Read the model definition and answer for the solid it produces. Units are mm, in the model's axes. Face numbers are marked on the shaded views. A direction names the side the tool comes from. Round coordinates to 2 decimals unless told otherwise and drop trailing zeros. Order: outer loops, then holes, each group sorted by start corner. A loop starts at its lowest first (then second) coordinate and runs counter-clockwise, first axis right, second up. Notation, with made-up numbers: (43.5, 75.25) -> (50.5, 75.25) arc R22 cw to (50.5, 84.25) -> close; hole circle Ø7 at (67, 86.25). An arc over 180 degrees is marked (long way). Use a Markdown table: item, result. Add a question column.
1. Section D-D, the plane x = 54.5 is taken. Give the vertices of the cut face in (y, z).
2. Given pin 1 (1.5 mm diameter, centred on y = 22, z = 5.5, fed in from +X); pin 2 (3.5 mm diameter, centred on x = -59.24, z = 0, fed in from +Y); pin 3 (2.5 mm diameter, centred on y = 131.5, z = 23, fed in from +X); pin 4 (2 mm diameter, centred on x = 0, z = 59.24, fed in from -Y), each flat-ended and moving along its own axis, determine where each tip first touches the part or whether it passes through.
3. Consider L1, parallel to Z at x = 0, y = 1; L2, parallel to Y at x = -34, z = -12; L3, parallel to Z at x = -13, y = 45.5. Determine where each line is inside the solid, lowest interval first. Write a range as [from, to].
4. Section A-A, the plane x = 7 is taken. Give the vertices of the cut face in (y, z), then the cut area to 3 significant figures.
5. Section C-C, the plane z = 18.5 is taken. Give the vertices of the cut face in (x, y), then the cut area to 3 significant figures.
6. Section B-B, the plane y = 11.5 is taken. Give the vertices of the cut face in (x, z).
7. For the marked faces 1 and 2, determine the directions among +Z, -Z, +X, -X, +Y, -Y from which every point of the face is accessible in a straight line to the end or side of a thin tool.
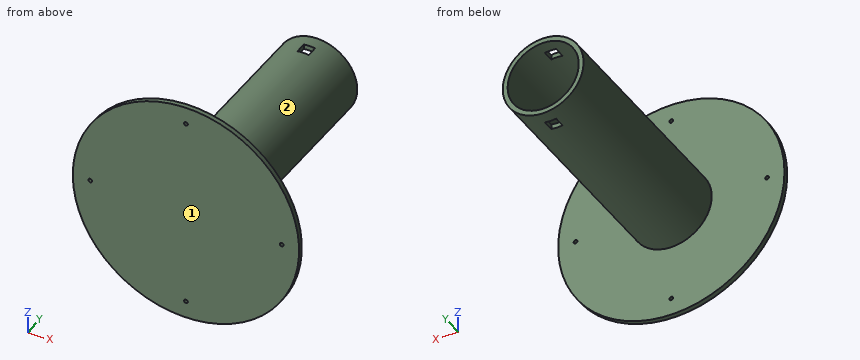
Autodesk Inventor part; units mm, degrees
ref_plane "YZ Plane" through (0, 0, 0) normal (1, 0, 0) x (0, 1, 0)
ref_plane "XZ Plane" through (0, 0, 0) normal (0, 1, 0) x (-1, 0, 0)
ref_plane "XY Plane" through (0, 0, 0) normal (0, 0, 1) x (1, 0, 0)
sketch "Sketch1" plane through (0, 0, 0) normal (0, 1, 0) x (-1, 0, 0)
  circle A0 centre (0, 0) radius 70
  dimension "d0" = 140
extrude "Extrusion1" add sketch "Sketch1" along normal blind 3
sketch "Sketch2" plane through (0, 3, 0) normal (0, 1, 0) x (1, 0, 0)
  circle A0 centre (0, 0) radius 25
  dimension "d3" = 50
extrude "Extrusion2" add sketch "Sketch2" along normal blind 140
shell "Shell1" thickness 3 removed faces 1 at (4.976, 143, 4.8639)
sketch "Sketch3" plane through (0, 3, 0) normal (0, 1, 0) x (1, 0, 0)
  circle A0 centre (0, 0) radius 25
  circle A1 centre (0, 0) radius 70
  circle A2 centre (0, 0) radius 70 construction
  line L0 (-70, 0) -> (70, 0) construction
  line L1 (0, 70) -> (0, -70) construction
  line L2 (0, 0) -> (-49.4975, -49.4975) construction
  line L3 (0, 0) -> (49.4975, -49.4975) construction
  point P0 (0, -59.2377)
  point P1 (0, 59.2377)
  point P2 (-59.2377, 0)
  point P3 (59.2377, 0)
  dimension "d14" = 45
  dimension "d15" = 45
hole "Hole1" at (0, 3, 59.2377) at (0, 3, -59.2377) at (59.2377, 3, 0) at (-59.2377, 3, 0) direction (0, -1, 0) diameter 2.3 end through all
sketch "Sketch4" plane through (0, 0, 0) normal (0, 0, 1) x (1, 0, 0)
  line L0 (25, 143) -> (-25, 143)
  line L1 (-25, 3) -> (25, 3)
  line L2 (70, 3) -> (-70, 3)
  line L3 (70, 0) -> (-70, 0)
  line L4 (25, 143) -> (-25, 143) construction
  line L5 (0, 143) -> (0, 0) construction
  line L6 (0, 143) -> (0, 0) construction
  line L7 (70, 3) -> (-70, 3) construction
  line L8 (-3.5, 135) -> (3.5, 135)
  line L9 (3.5, 135) -> (3.5, 128)
  line L10 (3.5, 128) -> (-3.5, 128)
  line L11 (-3.5, 128) -> (-3.5, 135)
  line L12 (-3.5, 135) -> (3.5, 128) construction
  line L13 (3.5, 135) -> (-3.5, 128) construction
  point P0 (0, 131.5)
  dimension "d18" = 7
  dimension "d19" = 7
  dimension "d23" = 125
extrude "Extrusion3" cut sketch "Sketch4" along normal mid plane 140
properties part number "bottom card holder"
Verdict:
| question | item | result |
|---|---|---|
| 1 | outline | (0, -43.93) -> (3, -43.93) -> (3, 43.93) -> (0, 43.93) -> close |
| 2 | pin 1 | stops at x = 24.54 |
| 2 | pin 2 | stops at y = 3 |
| 2 | pin 3 | stops at x = 12.33 |
| 2 | pin 4 | passes through |
| 3 | L1 | z = [-70, -60.39], [-58.09, 58.09], [60.39, 70] |
| 3 | L2 | y = [0, 3] |
| 3 | L3 | z = [-21.35, -17.75], [17.75, 21.35] |
| 4 | outline | (0, -69.65) -> (3, -69.65) -> (3, -24) -> (143, -24) -> (143, -20.86) -> (3, -20.86) -> (3, 20.86) -> (143, 20.86) -> (143, 24) -> (3, 24) -> (3, 69.65) -> (0, 69.65) -> close |
| 4 | area | 1,300 mm2 |
| 5 | outline | (-67.51, 0) -> (67.51, 0) -> (67.51, 3) -> (16.82, 3) -> (16.82, 143) -> (11.91, 143) -> (11.91, 3) -> (-11.91, 3) -> (-11.91, 143) -> (-16.82, 143) -> (-16.82, 3) -> (-67.51, 3) -> close |
| 5 | area | 1,780 mm2 |
| 6 | outline | circle Ø50 at (0, 0); hole circle Ø44 at (0, 0) |
| 7 | face 1 | +Z, -Z, +X, -X, -Y |
| 7 | face 2 | +Y |
